Input: part model. Units: mm. Frame: model coordinates. A direction names the side the tool comes from. Coordinates: 2 decimals unless noted, no trailing zeros. Write each loop counter-clockwise with the first axis right and the second up, starting at its lowest first coordinate (ties: lowest second). Pieces come first, ordered by that corner, then holes. Notation, with made-up numbers: (-10.75, -12.75) - (10.25, -12.75) arc R13 cw to (10.25, -3.75) - close; hole circle Ø4 at (-39, 16). An arc over 180 degrees is marked (long way). Use a Markdown table: item, result. Add a question column.
Q1. Set-up query: faces 1 (the face through (-120, 12, -2)), 2 (the face through (-61, 14, 33.608)), 3 (the face through (-5, 20, 22)). Return all of +Z, -Z, +X, -X, +Y, -Y with unobstructed straight access to the full face (end or side cutting, diameter ignored); none if empty.
Q2. Material intervals for probe 1 along Z at (x, y) = (-76.5, 21); probe 2 along X at (y, z) = (13.25, -11.5); probe 3 along Y at (x, z) = (-31, -5), sorted ascending. Write a range as from..to.
Q3. Mould query, pull axis Z, two halves, no side actions, for faces 4 (the face through (-59, 12, -46.392)), 5 (the face through (-110, 14, -2)), 6 (the face through (-5, 13, 11.608)), 7 (the face through (-59, 0, -1)). Classes: released by +Z, released by -Z, zero draft, split by the parting line, or undercut.
Q4. Pin query (flat end, axial travel): P1, Ø9, axis at x = -102.1, z = -27.73, coming from the -Y side; P2, Ø1.5, axis at x = -21, z = 26.5, coming from the +Y side. Return the tip coordinate at first contact, or that it passes through.
Q5. Section query D-D (y = 11.25). Return the cut outline in (x, z), then the cut area to 3 significant figures.
Q6. Section query C-C (z = 2). Return the cut outline in (x, y), then the cut area to 3 significant figures.
Q7. Section query B-B (x = -11.5). Return the cut outline in (y, z), then the cut area to 3 significant figures.
Q8. Section query A-A (y = 23). Return the cut outline in (x, z).
Autodesk Inventor part; units mm, degrees
ref_plane "YZ Plane" through (0, 0, 0) normal (1, 0, 0) x (0, 1, 0)
ref_plane "XZ Plane" through (0, 0, 0) normal (0, 1, 0) x (-1, 0, 0)
ref_plane "XY Plane" through (0, 0, 0) normal (0, 0, 1) x (1, 0, 0)
sketch "Sketch1" plane through (0, 0, 0) normal (0, 1, 0) x (-1, 0, 0)
  line L0 (120, 43.6082) -> (0, 43.6082)
  line L1 (0, 43.6082) -> (0, -46.3918)
  line L2 (0, -46.3918) -> (120, -46.3918)
  line L3 (120, -46.3918) -> (120, 43.6082)
  point P0 (0, 0)
  dimension "d0" = 90
  dimension "d1" = 120
  dimension "d2" = 0
extrude "Extrusion1" add sketch "Sketch1" along normal blind 25
sketch "Sketch2" plane through (0, 25, 0) normal (0, 1, 0) x (1, 0, 0)
  line L0 (-110, -33.6082) -> (-10, -33.6082)
  line L1 (-10, -33.6082) -> (-10, 36.3918)
  line L2 (-10, 36.3918) -> (-110, 36.3918)
  line L3 (-110, 36.3918) -> (-110, -33.6082)
  line L4 (-120, -43.6082) -> (0, -43.6082)
  line L5 (0, 46.3918) -> (-120, 46.3918)
  line L6 (-120, 46.3918) -> (-120, -43.6082)
  line L7 (0, -43.6082) -> (0, 46.3918)
  point P0 (0, 0)
  dimension "d5" = 10
  dimension "d6" = 10
  dimension "d7" = 10
  dimension "d8" = 10
extrude "Extrusion2" cut sketch "Sketch2" against normal blind 22 contours L3 L2 L1 L0
sketch "Sketch4" plane through (0, 0, 43.6082) normal (1, 0, 0) x (0, 0, -1)
  line L0 (12, 20) -> (32, 20)
  line L1 (32, 20) -> (32, 5)
  line L2 (32, 5) -> (12, 5)
  line L3 (12, 5) -> (12, 20)
  line L4 (0, 25) -> (90, 25)
  line L5 (0, 0) -> (90, 0)
  line L6 (90, 0) -> (90, 25)
  line L7 (0, 0) -> (0, 25)
  point P0 (43.6082, 0)
  dimension "d13" = 5
  dimension "d14" = 5
  dimension "d16" = 20
  dimension "d19" = 12
extrude "Extrusion3" cut sketch "Sketch4" against normal blind 22 contours L0 L1 L2 L3
sketch "Sketch5" plane through (0, 3, 0) normal (0, 1, 0) x (1, 0, 0)
  circle A0 centre (-102.0989, 27.7281) radius 4.8843
  line L0 (-110, -33.6082) -> (-110, 36.3918)
  line L1 (-110, 36.3918) -> (-10, 36.3918)
  point P0 (0, 0)
  dimension "d20" = 7.9011
  dimension "d21" = 8.6636
extrude "Extrusion4" cut sketch "Sketch5" against normal blind 22
properties part number "Case_Bottom_Part"
Values follow:
| question | item | result |
|---|---|---|
| 1 | face 1 | +Z, -Z, -X, +Y, -Y |
| 1 | face 2 | +Y |
| 1 | face 3 | +X |
| 2 | probe 1 | -46.39..-36.39, 33.61..43.61 |
| 2 | probe 2 | -120..-110, -10..0 |
| 2 | probe 3 | 0..3 |
| 3 | face 4 | released by -Z |
| 3 | face 5 | undercut |
| 3 | face 6 | undercut |
| 3 | face 7 | zero draft |
| 4 | P1 | through |
| 4 | P2 | y = 3 |
| 5 | outline | (-120, -46.39) - (0, -46.39) - (0, 11.61) - (-10, 11.61) - (-10, -36.39) - (-110, -36.39) - (-110, 33.61) - (-10, 33.61) - (-10, 31.61) - (0, 31.61) - (0, 43.61) - (-120, 43.61) - close |
| 5 | area | 3,600 mm2 |
| 6 | outline | (-120, 0) - (0, 0) - (0, 25) - (-10, 25) - (-10, 3) - (-110, 3) - (-110, 25) - (-120, 25) - close |
| 6 | area | 800 mm2 |
| 7 | outline | (0, -46.39) - (25, -46.39) - (25, -36.39) - (3, -36.39) - (3, 33.61) - (25, 33.61) - (25, 43.61) - (0, 43.61) - close |
| 7 | area | 710 mm2 |
| 8 | outline | (-120, -46.39) - (0, -46.39) - (0, 43.61) - (-120, 43.61) - close; hole (-110, -36.39) - (-10, -36.39) - (-10, 33.61) - (-110, 33.61) - close |
